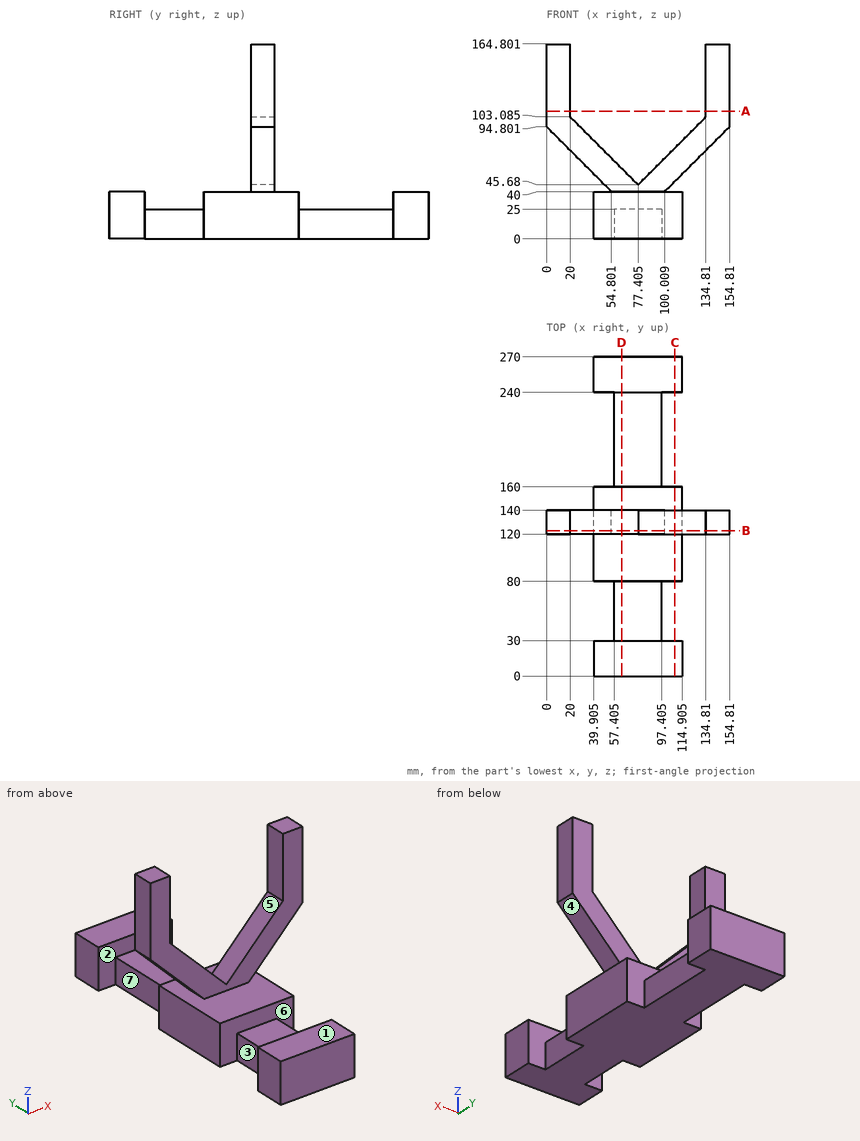
For this review, use the dimensioned drawing (mm, ordinates from the lowest corner) and the shaded views. A direction names the side the tool comes from. Round coordinates to 2 decimals unless told otherwise and drop trailing zeros. Write each loop counter-clockwise with the first axis right and the second up, starting at its lowest first coordinate (ties: lowest second). Pieces come first, ordered by that corner, then holes. Notation, with made-up numbers: M 28,16 L 84,16 A23 cw 84,43 Z; hole C 46,-33.75 d10. An arc over 180 degrees is marked long. Use CSV: the item, a comma, the result in double quotes. Start each with the question number.
(1) The part is to be moulded in two halves that separate along X. For the marked faces 5, 6 and 7, say which applies: +X half, -X half, draft (parallel to the pull), parting line (faces both ways), or undercut.
(2) We need section A-A, the plane z = 108. State the section outline as (x, y) points.
(3) We need section B-B, the plane y = 123. State the section outline as (x, z) points (1 decimal).
(4) We need section C-C, the plane x = 108.5. State the section outline as (y, z) points (1 decimal), then the cut area to 3 significant figures.
(5) We need section D-D, the plane x = 63.5. State the section outline as (y, z) points (1 decimal), then the cut area to 3 significant figures.
(6) Tool access review of the marked faces 1, 2, 3 and 4: name each direction out of +Z, -Z, +X, -X, +Y, -Y from which nothing blocks a thin tool from reaching the whole face with its end or side.
(7) For line 1 along Z through (x, y) = (106, 116); line 2 along Z through (x, y) = (96, 180); line 3 along Y through (x, z) = (135, 146.5), list the stretches that pass through material, from the lowest coordinate up.
(8) Clearance check with flat-ended pins moving along their axes: P1, Ø20, axis at y = 187, z = 7, coming from the +X side (3 decimals); P2, Ø9, axis at x = 88.5, y = 254, coming from the +Z side; P3, Ø15, axis at y = 20.5, z = 21, coming from the -X side (3 decimals); P4, Ø10, axis at x = 123, z = 30.5, coming from the +Y side. State where each tip first meets the part, or that it passes through.
Findings:
1,face 5,"undercut"
1,face 6,"draft"
1,face 7,"-X half"
2,outline,"M 0,120 L 20,120 L 20,140 L 0,140 Z; M 134.81,120 L 154.81,120 L 154.81,140 L 134.81,140 Z"
3,outline,"M 0,94.8 L 54.8,40 L 39.9,40 L 39.9,0 L 114.9,0 L 114.9,40 L 100,40 L 154.8,94.8 L 154.8,164.8 L 134.8,164.8 L 134.8,103.1 L 77.4,45.7 L 20,103.1 L 20,164.8 L 0,164.8 Z"
4,outline,"M 0,0 L 30,0 L 30,40 L 0,40 Z; M 80,0 L 160,0 L 160,40 L 80,40 Z; M 120,48.5 L 140,48.5 L 140,76.8 L 120,76.8 Z; M 240,0 L 270,0 L 270,40 L 240,40 Z"
4,area,"6,170 mm^2"
5,outline,"M 0,0 L 270,0 L 270,40 L 240,40 L 240,25 L 160,25 L 160,40 L 140,40 L 140,59.6 L 120,59.6 L 120,40 L 80,40 L 80,25 L 30,25 L 30,40 L 0,40 Z"
5,area,"9,240 mm^2"
6,face 1,"+Z, +X, -X, -Y"
6,face 2,"+Z"
6,face 3,"+Z, -Z, -X"
6,face 4,"+X, +Y, -Y"
7,line 1,"0 to 40"
7,line 2,"0 to 25"
7,line 3,"120 to 140"
8,P1,"x = 97.405"
8,P2,"z = 40"
8,P3,"x = 39.905"
8,P4,"through"
